Geometry check sheet. Reference: drawing and pictorial views, mm from the part's lowest x, y, z. Round coordinates to 2 decimals unless told otherwise and drop trailing zeros. Order: outer loops, then holes, each group sorted by start corner. A loop starts at its lowest first (then second) coordinate and runs counter-clockwise, first axis right, second up.
(1) Thickness scan on L1, parallel to Y at x = 14.5, z = 0.7; L2, parallel to Y at x = 18.25, z = 3; L3, parallel to Y at x = 23, z = 1.1. Record the ranges inside material, lowest first.
(2) Cross-section at A-A on y = 37. Enter the section's corners in (x, z).
(3) Cross-section at D-D on y = 44.5. Enter the section's corners in (x, z).
(4) Gauge pin test, flat end, axial feed: P1, Ø3, axis at x = 16.5, y = 37, coming from the -Z side (1 decimal). Record the tip position at first contact, or that the pin passes through.
(5) Cross-section at C-C on y = 11.5. Enter the section's corners in (x, z), and give its area (3 significant figures).
(6) Cross-section at B-B on z = 0.75. Enter the section's corners in (x, y).
(7) Draft check along X on the marked faces 1, 2, 3 and 4. Enter one of: pulls with the +X half, pulls with the -X half, needs draft (parallel to the pull), parting line crosses it, or undercut.
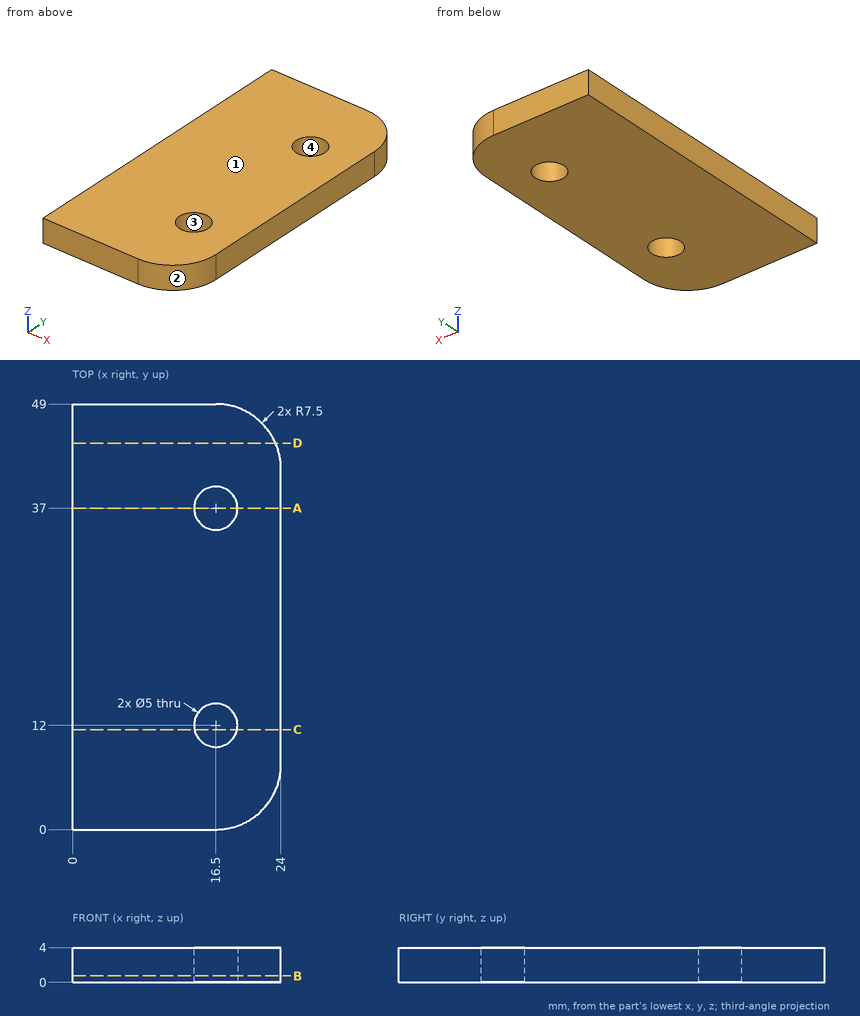
Found:
1. L1: y = 0 to 10.5, 13.5 to 35.5, 38.5 to 49
1. L2: y = 0.21 to 10.21, 13.79 to 35.21, 38.79 to 48.79
1. L3: y = 3.76 to 45.24
2. outline: (0, 0) - (14, 0) - (14, 4) - (0, 4) - close; (19, 0) - (24, 0) - (24, 4) - (19, 4) - close
3. outline: (0, 0) - (23.37, 0) - (23.37, 4) - (0, 4) - close
4. P1: passes through
5. outline: (0, 0) - (14.05, 0) - (14.05, 4) - (0, 4) - close; (18.95, 0) - (24, 0) - (24, 4) - (18.95, 4) - close
5. area: 76.4 mm2
6. outline: (0, 0) - (16.5, 0) arc R7.5 ccw to (24, 7.5) - (24, 41.5) arc R7.5 ccw to (16.5, 49) - (0, 49) - close; hole circle Ø5 at (16.5, 12); hole circle Ø5 at (16.5, 37)
7. face 1: needs draft
7. face 2: pulls with the +X half
7. face 3: undercut
7. face 4: undercut
